```python
from build123d import *

# Parameters (mm, degrees)
SKETCH1_W           = 215.28
SKETCH1_H           = 157.9
SKETCH1_R           = 2.3
BOSS_EXTRUDE1_DEPTH = 7.5
SKETCH1_2_R         = 2.3
BOSS_EXTRUDE2_DEPTH = 2
CUT_EXTRUDE1_DEPTH  = 3.5
SKETCH3_W           = 16
SKETCH3_H           = 60
SKETCH3_W_2         = 40
SKETCH3_H_2         = 16
BOSS_EXTRUDE3_DEPTH = 7.5
FILLET1_R           = 0.5
FILLET2_R           = 3


with BuildPart() as part:
    # Sketch1 → Boss-Extrude1 (new body)
    with BuildSketch(Plane(origin=(0, 0, 0), x_dir=(1, 0, 0), z_dir=(0, 1, 0))):
        with Locations((104.14, 75.45)):
            Rectangle(SKETCH1_W, SKETCH1_H)
        with Locations((5.5, 145.4)):
            Circle(SKETCH1_R, mode=Mode.SUBTRACT)
        with Locations((5.5, 7)):
            Circle(SKETCH1_R, mode=Mode.SUBTRACT)
        with Locations((200.78, 7)):
            Circle(SKETCH1_R, mode=Mode.SUBTRACT)
        with Locations((200.78, 145.4)):
            Circle(SKETCH1_R, mode=Mode.SUBTRACT)
    extrude(amount=BOSS_EXTRUDE1_DEPTH)

    # Sketch1<2> → Boss-Extrude2 (add)
    with BuildSketch(Plane(origin=(0, 0, 0), x_dir=(1, 0, 0), z_dir=(0, 1, 0))):
        with Locations((200.78, 145.4)):
            Circle(SKETCH1_2_R)
        with Locations((5.5, 7)):
            Circle(SKETCH1_2_R)
        with Locations((5.5, 145.4)):
            Circle(SKETCH1_2_R)
        with Locations((200.78, 7)):
            Circle(SKETCH1_2_R)
    extrude(amount=BOSS_EXTRUDE2_DEPTH)

    # Sketch2 → Cut-Extrude1 (cut)
    with BuildSketch(Plane(origin=(0, 7.5, 0), x_dir=(1, 0, 0), z_dir=(0, 1, 0))):
        with BuildLine():
            Line((21.303480629, 150.9), (184.976519371, 150.9))
            ThreePointArc((184.976519371, 150.9), (190.172671793, 148.98276253), (192.878259685, 144.15))
            ThreePointArc((192.878259685, 144.15), (195.123145751, 139.743145751), (199.53, 137.498259685))
            ThreePointArc((199.53, 137.498259685), (204.36276253, 134.792671793), (206.28, 129.596519371))
            Line((206.28, 129.596519371), (206.28, 22.803480629))
            ThreePointArc((206.28, 22.803480629), (204.36276253, 17.607328207), (199.53, 14.901740315))
            ThreePointArc((199.53, 14.901740315), (194.862670388, 12.383791439), (192.795640289, 7.5))
            ThreePointArc((192.795640289, 7.5), (190.288506152, 2.169048105), (184.811280577, 0))
            Line((184.811280577, 0), (21.468719423, 0))
            ThreePointArc((21.468719423, 0), (15.991493848, 2.169048105), (13.484359711, 7.5))
            ThreePointArc((13.484359711, 7.5), (11.417329612, 12.383791439), (6.75, 14.901740315))
            ThreePointArc((6.75, 14.901740315), (1.91723747, 17.607328207), (0, 22.803480629))
            Line((0, 22.803480629), (0, 129.596519371))
            ThreePointArc((0, 129.596519371), (1.91723747, 134.792671793), (6.75, 137.498259685))
            ThreePointArc((6.75, 137.498259685), (11.156854249, 139.743145751), (13.401740315, 144.15))
            ThreePointArc((13.401740315, 144.15), (16.107328207, 148.98276253), (21.303480629, 150.9))
        make_face()
    extrude(amount=-CUT_EXTRUDE1_DEPTH, mode=Mode.SUBTRACT)

    # Sketch3 → Boss-Extrude3 (add)
    with BuildSketch(Plane(origin=(0, 7.5, 0), x_dir=(1, 0, 0), z_dir=(0, 1, 0))):
        with Locations((-11.5, 26.5)):
            Rectangle(SKETCH3_W, SKETCH3_H)
        with BuildLine():
            Line((-8.25, 48.75), (-8.25, 4.25))
            ThreePointArc((-8.25, 4.25), (-11.5, 1), (-14.75, 4.25))
            Line((-14.75, 4.25), (-14.75, 48.75))
            ThreePointArc((-14.75, 48.75), (-11.5, 52), (-8.25, 48.75))
        make_face(mode=Mode.SUBTRACT)
        with Locations((16.5, 162.4)):
            Rectangle(SKETCH3_W_2, SKETCH3_H_2)
        with BuildLine():
            Line((4.25, 165.65), (28.75, 165.65))
            ThreePointArc((28.75, 165.65), (32, 162.4), (28.75, 159.15))
            Line((28.75, 159.15), (4.25, 159.15))
            ThreePointArc((4.25, 159.15), (1, 162.4), (4.25, 165.65))
        make_face(mode=Mode.SUBTRACT)
        with Locations((191.78, 162.4)):
            Rectangle(SKETCH3_W_2, SKETCH3_H_2)
        with BuildLine():
            Line((179.53, 165.65), (204.03, 165.65))
            ThreePointArc((204.03, 165.65), (207.28, 162.4), (204.03, 159.15))
            Line((204.03, 159.15), (179.53, 159.15))
            ThreePointArc((179.53, 159.15), (176.28, 162.4), (179.53, 165.65))
        make_face(mode=Mode.SUBTRACT)
    extrude(amount=-BOSS_EXTRUDE3_DEPTH)

    # Fillet1
    fillet1_edges = [part.edges().sort_by_distance(p)[0] for p in [
        (190.288506152, 7.5, -2.169048105),
        (194.862670388, 7.5, -12.383791439),
        (204.36276253, 7.5, -17.607328207),
        (206.28, 7.5, -76.2),
        (204.36276253, 7.5, -134.792671793),
        (195.123145751, 7.5, -139.743145751),
        (190.172671793, 7.5, -148.98276253),
        (103.14, 7.5, -150.9),
        (16.107328207, 7.5, -148.98276253),
        (11.156854249, 7.5, -139.743145751),
        (1.91723747, 7.5, -134.792671793),
        (0, 7.5, -76.2),
        (1.91723747, 7.5, -17.607328207),
        (11.417329612, 7.5, -12.383791439),
        (15.991493848, 7.5, -2.169048105),
        (103.14, 7.5, 0),
    ]]
    fillet(fillet1_edges, radius=FILLET1_R)

    # Fillet2
    fillet2_edges = [part.edges().sort_by_distance(p)[0] for p in [
        (-19.5, 3.75, -56.5),
        (-3.5, 3.75, -170.4),
        (36.5, 3.75, -170.4),
        (36.5, 3.75, -154.4),
        (211.78, 3.75, -170.4),
        (171.78, 3.75, -154.4),
        (171.78, 3.75, -170.4),
        (211.78, 3.75, 3.5),
        (-3.5, 3.75, -56.5),
        (-19.5, 3.75, 3.5),
    ]]
    fillet(fillet2_edges, radius=FILLET2_R)


solid = part.part
```
Input: part model. Units: mm. Frame: model coordinates. A direction names the side the tool comes from. Coordinates: 2 decimals unless noted, no trailing zeros. Write each loop counter-clockwise with the first axis right and the second up, starting at its lowest first coordinate (ties: lowest second). Pieces come first, ordered by that corner, then holes. Notation, with made-up numbers: M -14,28.25 L -10,28.25 A28 cw -10,47.25 Z; hole C 74.5,65.25 d4. An arc over 180 degrees is marked long. Use one line per item in the form item = value.
Q1. Set-up query: faces 1 (the face through (-11.4, 3.8, -1)), 2 (the face through (-3.5, 4, -113)), 3 (the face through (95, 4, 3.5)), 4 (the face through (5, 2, -145)). Return all of +Z, -Z, +X, -X, +Y, -Y with unobstructed straight access to the full face (end or side cutting, diameter ignored); none if empty.
Answer below:
face_1 = +Y, -Y
face_2 = -Z, -X, +Y, -Y
face_3 = +Z, +X, -X, +Y, -Y
face_4 = +Y
Q2. Section A-A (x = -11.5). Return loops of the section in (y, z), plus the area to 3 significant figures.
Answer below:
outline = M 0,-56.5 L 7.5,-56.5 L 7.5,-52 L 0,-52 Z; M 0,-1 L 7.5,-1 L 7.5,3.5 L 0,3.5 Z
area = 67.5 mm²
Q3. Draft query along X for faces 5 (the face through (16, 4, -165.65)), 6 (the face through (211.78, 4, -82)), 7 (the face through (16, 4, -170.4)). Return one class per face: released by +X, released by -X, zero draft, split by the parting line, or undercut.
Answer below:
face_5 = undercut
face_6 = released by +X
face_7 = zero draft
Q4. Material intervals for probe 1 along X at (y, z) = (3.35, -7); probe 2 along X at (y, z) = (5.2, -7); probe 3 along X at (y, z) = (3.2, -145.4), sorted ascending. Write a range as from..to.
Answer below:
probe_1 = -19.5..-14.75, -8.25..3.2, 7.8..198.48, 203.08..211.78
probe_2 = -19.5..-14.75, -8.25..3.2, 7.8..13.53, 192.75..198.48, 203.08..211.78
probe_3 = -3.5..3.2, 7.8..198.48, 203.08..211.78
Q5. Section B-B (z = -81). Return loops of the section in (x, y), plus the area to 3 significant figures.
Answer below:
outline = M -3.5,0 L 211.78,0 L 211.78,7.5 L 206.78,7.5 A0.5 ccw 206.28,7 L 206.28,4 L 0,4 L 0,7 A0.5 ccw -0.5,7.5 L -3.5,7.5 Z
area = 893 mm²
Q6. First-contact query: pin 1 (3.5 mm diameter, centred on x = 200.78, z = -145.4, fed in from +Y); pin 2 (4 mm diameter, centred on y = 2.5, z = -161.5, fed in from -X); pin 3 (1.5 mm diameter, centred on x = 116, z = -70, fed in from +Y). Flat tips, straight axial feed; report the tip coordinate or a pass-through.
Answer below:
pin_1 = 2
pin_2 = -3.5
pin_3 = 4
Q7. Section C-C (x = 113.5). Return loops of the section in (y, z).
Answer below:
outline = M 0,-154.4 L 7.5,-154.4 L 7.5,-151.4 A0.5 ccw 7,-150.9 L 4,-150.9 L 4,0 L 7,0 A0.5 ccw 7.5,0.5 L 7.5,3.5 L 0,3.5 Z
